```python
from build123d import *

# Parameters (mm, degrees)
BOSS_EXTRUDE1_DEPTH     = 31.75
SHELL1_T                = -7.62
SKETCH1_5_W             = 101.6
SKETCH1_5_H             = 50.8
BOSS_EXTRUDE3_DEPTH     = 19.05
CUT_EXTRUDE2_DEPTH      = 506.280856772
CUT_EXTRUDE2_DEPTH_BACK = 506.280856772
SKETCH4_W               = 63.5
SKETCH4_H               = 50.8
FILLET5_R               = 7.62
FILLET6_R               = 5.08
FILLET7_R               = 7.62
FILLET8_R               = 5.08
FILLET9_R               = 5.08
FILLET10_R              = 5.08
FILLET11_R              = 2.54
FILLET12_R              = 2.54
FILLET13_R              = 2.54
FILLET14_R              = 2.54
CUT_EXTRUDE3_DEPTH      = 406.583478584
CUT_EXTRUDE3_DEPTH_BACK = 406.583478584
SKETCH5_R               = 2.54


with BuildPart() as part:
    # Sketch1 → Boss-Extrude1 (new body)
    with BuildSketch(Plane(origin=(0, 0, 0), x_dir=(1, 0, 0), z_dir=(0, 1, 0))):
        with BuildLine():
            Line((0, 260.9596), (381, 260.9596))
            ThreePointArc((381, 260.9596), (392.440846298, 256.220646298), (397.1798, 244.7798))
            Line((397.1798, 244.7798), (397.1798, 16.1798))
            ThreePointArc((397.1798, 16.1798), (392.440846298, 4.738953702), (381, 0))
            Line((381, 0), (0, 0))
            ThreePointArc((0, 0), (-11.440846298, 4.738953702), (-16.1798, 16.1798))
            Line((-16.1798, 16.1798), (-16.1798, 244.7798))
            ThreePointArc((-16.1798, 244.7798), (-11.440846298, 256.220646298), (0, 260.9596))
        make_face()
    extrude(amount=BOSS_EXTRUDE1_DEPTH)

    # Shell1
    shell1_openings = [part.faces().sort_by_distance(p)[0] for p in [
        (190.5, 0, -130.4798),
    ]]
    offset(amount=SHELL1_T, openings=shell1_openings, kind=Kind.INTERSECTION)

    # Sketch1_5 → Boss-Extrude3 (add)
    with BuildSketch(Plane(origin=(0, 0, 0), x_dir=(1, 0, 0), z_dir=(0, 1, 0))):
        with Locations((190.5, 286.3596)):
            Rectangle(SKETCH1_5_W, SKETCH1_5_H)
    extrude(amount=BOSS_EXTRUDE3_DEPTH)

    # Sketch4 → Cut-Extrude2 (cut, two sides: drawn at the far end of the back side and taken through both)
    with BuildSketch(Plane(origin=(0, 19.05, 0), x_dir=(1, 0, 0), z_dir=(0, 1, 0)).offset(-CUT_EXTRUDE2_DEPTH_BACK)):
        with Locations((190.5, 286.3596)):
            Rectangle(SKETCH4_W, SKETCH4_H)
    extrude(amount=CUT_EXTRUDE2_DEPTH + CUT_EXTRUDE2_DEPTH_BACK, mode=Mode.SUBTRACT)

    # Fillet5
    fillet5_edges = [part.edges().sort_by_distance(p)[0] for p in [
        (231.775, 19.05, -311.7596),
    ]]
    fillet(fillet5_edges, radius=FILLET5_R)

    # Fillet6
    fillet6_edges = [part.edges().sort_by_distance(p)[0] for p in [
        (231.775, 0, -311.7596),
    ]]
    fillet(fillet6_edges, radius=FILLET6_R)

    # Fillet7
    fillet7_edges = [part.edges().sort_by_distance(p)[0] for p in [
        (149.225, 19.05, -311.7596),
    ]]
    fillet(fillet7_edges, radius=FILLET7_R)

    # Fillet8
    fillet8_edges = [part.edges().sort_by_distance(p)[0] for p in [
        (149.225, 0, -311.7596),
    ]]
    fillet(fillet8_edges, radius=FILLET8_R)

    # Fillet9
    fillet9_edges = [part.edges().sort_by_distance(p)[0] for p in [
        (231.775, 19.05, -260.9596),
    ]]
    fillet(fillet9_edges, radius=FILLET9_R)

    # Fillet10
    fillet10_edges = [part.edges().sort_by_distance(p)[0] for p in [
        (149.225, 19.05, -260.9596),
    ]]
    fillet(fillet10_edges, radius=FILLET10_R)

    # Fillet11
    fillet11_edges = [part.edges().sort_by_distance(p)[0] for p in [
        (241.3, 12.065, -260.9596),
    ]]
    fillet(fillet11_edges, radius=FILLET11_R)

    # Fillet12
    fillet12_edges = [part.edges().sort_by_distance(p)[0] for p in [
        (222.25, 12.065, -260.9596),
    ]]
    fillet(fillet12_edges, radius=FILLET12_R)

    # Fillet13
    fillet13_edges = [part.edges().sort_by_distance(p)[0] for p in [
        (158.75, 12.065, -260.9596),
    ]]
    fillet(fillet13_edges, radius=FILLET13_R)

    # Fillet14
    fillet14_edges = [part.edges().sort_by_distance(p)[0] for p in [
        (139.7, 12.065, -260.9596),
    ]]
    fillet(fillet14_edges, radius=FILLET14_R)

    # Sketch5 → Cut-Extrude3 (cut, two sides: drawn at the far end of the back side and taken through both)
    with BuildSketch(Plane(origin=(241.3, 0, 0), x_dir=(0, 0, -1), z_dir=(1, 0, 0)).offset(-CUT_EXTRUDE3_DEPTH_BACK)):
        with Locations((301.5996, 9.525)):
            Circle(SKETCH5_R)
        with Locations((281.2796, 9.525)):
            Circle(SKETCH5_R)
    extrude(amount=CUT_EXTRUDE3_DEPTH + CUT_EXTRUDE3_DEPTH_BACK, mode=Mode.SUBTRACT)


solid = part.part
```
The listing builds one solid part. Answer for the finished solid, in the listing's coordinates (mm). A direction names the side the tool comes from. Round coordinates to 2 decimals unless told otherwise and drop trailing zeros. Loops run counter-clockwise (first coordinate to the right, second up) from the corner with the lowest first, then second, coordinate; pieces in that order, holes last.
Q1. Find the intervals of material crossed by line 1 (X direction, y = 17, z = -29); line 2 (Z direction, x = 98, y = 11); line 3 (Y direction, x = 88, z = -60), in increasing order.
Q2. Which of the six approach directions +Z, -Z, +X, -X, +Y, -Y give full straight-line access (tool end or side, diameter ignored) to faces 4 (the face through (139.7, 10, -287)), 5 (the face through (241.3, 10, -287)), 6 (the face through (149, 19.05, -285)), 7 (the face through (237, 0, -256)), 8 (the face through (-6.119, 11.896, -250.766))?
Q3. For a pull along Z with two mould halves and no side action, classify faces 1 (the face through (-11.57, 15.65, -256.09)), 2 (the face through (222.25, 10, -287)), 3 (the face through (387.119, 11.896, -10.194)) as released by +Z, released by -Z, zero draft, split by the parting line, or undercut.
Q4. Section A-A, the plane z = -31 is taken. Determine the outline of the cut face in (x, y).
Q5. Given pin 1 Ø2 at (x, y) = (190, 14.5) entering from -Z; pin 2 Ø4 at (x, z) = (120.5, -109) entering from -Y; pin 3 Ø6 at (y, z) = (9.52, -281.28) entering from -X; pin 4 Ø4.5 at (y, z) = (9.52, -301.6) entering from +X, each flat-ended and moving along its own axis, determine where each tip first touches the part or whether it passes through.
Q6. Section C-C, the plane x = 145 is taken. Determine the outline of the cut face in (y, z) (3 decimals).
Q7. Section B-B, the plane x = 200 is taken. Determine the outline of the cut face in (y, z).
Completed:
1. line 1: x = -16.18 to -8.56, 389.56 to 397.18
1. line 2: z = -260.96 to -253.34, -7.62 to 0
1. line 3: y = 24.13 to 31.75
2. face 4: -Z, -X, +Y, -Y
2. face 5: -Z, +X, +Y, -Y
2. face 6: -Z, +X, -X, +Y
2. face 7: +Z, -Z, +X, -X, -Y
2. face 8: -Y
3. face 1: released by -Z
3. face 2: zero draft
3. face 3: undercut
4. outline: (-16.18, 0) - (-8.56, 0) - (-8.56, 24.13) - (389.56, 24.13) - (389.56, 0) - (397.18, 0) - (397.18, 31.75) - (-16.18, 31.75) - close
5. pin 1: stops at z = -260.96
5. pin 2: stops at y = 24.13
5. pin 3: stops at x = 139.7
5. pin 4: passes through
6. outline: (0, -306.68) arc R5.08 ccw to (5.08, -311.76) - (11.43, -311.76) arc R7.62 ccw to (19.05, -304.14) - (19.05, -266.04) arc R5.08 cw to (24.13, -260.96) - (31.75, -260.96) - (31.75, 0) - (0, 0) - (0, -7.62) - (24.13, -7.62) - (24.13, -253.34) - (0, -253.34) - close; hole circle Ø5.08 at (9.525, -301.6); hole circle Ø5.08 at (9.525, -281.28)
7. outline: (0, -260.96) - (31.75, -260.96) - (31.75, 0) - (0, 0) - (0, -7.62) - (24.13, -7.62) - (24.13, -253.34) - (0, -253.34) - close
